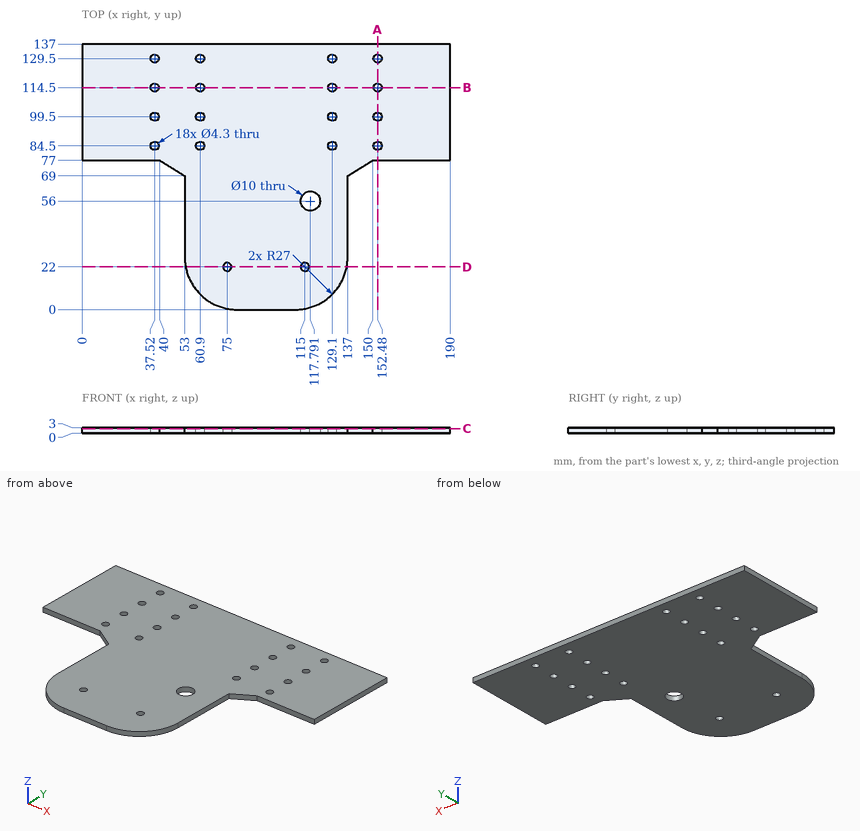
Drawing for the job (mm, zero at the part's lowest x, y, z). Round coordinates to 2 decimals unless told otherwise and drop trailing zeros. Loops run counter-clockwise (first coordinate to the right, second up) from the corner with the lowest first, then second, coordinate; pieces in that order, holes last.
1. Band-saw the part on C-C, the plane z = 2.5. Count the separate pieces of the cut face and the enclosed holes in it, and give its area (3 significant figures).
Check values:
separate pieces: 1
enclosed holes: 19
area: 17,300 mm2
2. Band-saw the part on D-D, the plane y = 22. List the corners of the cut face in (x, z).
Check values:
outline: (53.47, 0) - (72.85, 0) - (72.85, 3) - (53.47, 3) - close; (77.15, 0) - (112.85, 0) - (112.85, 3) - (77.15, 3) - close; (117.15, 0) - (136.53, 0) - (136.53, 3) - (117.15, 3) - close
3. Wall check: probe 1 along X at (y, z) = (129.5, 1.25); probe 2 along Y at (x, z) = (152.48, 1.35); probe 3 along Y at (x, z) = (129.1, 1.4). Give the ranges that are in metal, low to high.
Check values:
probe 1: x = 0 to 35.37, 39.67 to 58.75, 63.05 to 126.95, 131.25 to 150.33, 154.63 to 190
probe 2: y = 77 to 82.35, 86.65 to 97.35, 101.65 to 112.35, 116.65 to 127.35, 131.65 to 137
probe 3: y = 7.92 to 82.35, 86.65 to 97.35, 101.65 to 112.35, 116.65 to 127.35, 131.65 to 137
4. Drop flat-ended pins along their axis: P1, Ø5, axis at x = 152.48, y = 114.5, coming from the -Z side; P2, Ø0.9, axis at x = 14.5, z = 1.5, coming from the -Y side; P3, Ø0.9, axis at y = 42.5, z = 1.5, coming from the -X side. Give the stop position or say it passes through.
Check values:
P1: stops at z = 0
P2: stops at y = 77
P3: stops at x = 53
5. Band-saw the part on A-A, the plane x = 152.48. List the corners of the cut face in (y, z).
Check values:
outline: (77, 0) - (82.35, 0) - (82.35, 3) - (77, 3) - close; (86.65, 0) - (97.35, 0) - (97.35, 3) - (86.65, 3) - close; (101.65, 0) - (112.35, 0) - (112.35, 3) - (101.65, 3) - close; (116.65, 0) - (127.35, 0) - (127.35, 3) - (116.65, 3) - close; (131.65, 0) - (137, 0) - (137, 3) - (131.65, 3) - close
6. Band-saw the part on B-B, the plane y = 114.5. List the corners of the cut face in (x, z).
Check values:
outline: (0, 0) - (35.37, 0) - (35.37, 3) - (0, 3) - close; (39.67, 0) - (58.75, 0) - (58.75, 3) - (39.67, 3) - close; (63.05, 0) - (126.95, 0) - (126.95, 3) - (63.05, 3) - close; (131.25, 0) - (150.33, 0) - (150.33, 3) - (131.25, 3) - close; (154.63, 0) - (190, 0) - (190, 3) - (154.63, 3) - close
